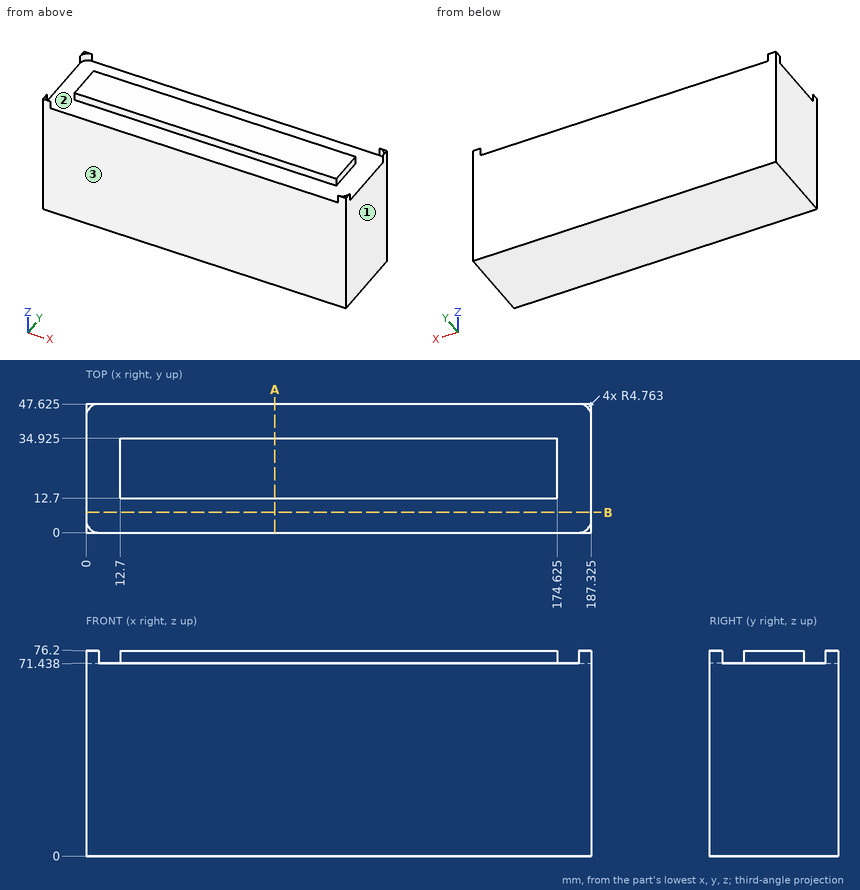
Here's the drawing with two shaded views (mm, measured from the low corner). I have some questions. Round coordinates to 2 decimals unless told otherwise and drop trailing zeros. Loops run counter-clockwise (first coordinate to the right, second up) from the corner with the lowest first, then second, coordinate; pieces in that order, holes last. Notation, with made-up numbers: M 51.25,66.5 L 103.25,66.5 A19 ccw 103.25,91.5 Z; hole C -22.75,5.25 d1. An arc over 180 degrees is marked long. Answer as a JSON object with one key per item and string values. Group by question number.
Q1. Imagine slicing it at B-B, the plane y = 7.5. Please give me the cut outline in (x, z) (1 decimal).
Q2. We'd pull the mould along X, two halves only. Please class the marked faces 1, 2 and 3: +X half, -X half, draft (parallel to the pull), parting line (faces both ways), or undercut.
Q3. Will these pins go through, and if not, where does the flat tip stop? pin 1 (5 mm diameter, centred on y = 23, z = 73.5, fed in from +X) (1 decimal); pin 2 (1.4 mm diameter, centred on x = 113, z = 74, fed in from +Y) (1 decimal); pin 3 (6 mm diameter, centred on x = 82.5, y = 40, fed in from +Z); pin 4 (2.5 mm diameter, centred on x = 118, z = 74.5, fed in from -Y).
Q4. Please list where this line runs through material, in increasing order: L1, parallel to Z at x = 148.5, y = 44.
Q5. Imagine slicing it at A-A, the plane x = 70. Please give me the cut outline in (y, z) (1 decimal), then the cut area to 3 significant figures.
Findings:
{
 "1": {"outline": "M 0,0 L 187.3,0 L 187.3,71.4 L 0,71.4 Z"},
 "2": {"face 1": "+X half", "face 2": "undercut", "face 3": "draft"},
 "3": {"pin 1": "stops at x = 187.3", "pin 2": "stops at y = 34.9", "pin 3": "stops at z = 71.44", "pin 4": "stops at y = 12.7"},
 "4": {"L1": "z = 0 to 71.44"},
 "5": {"outline": "M 0,0 L 47.6,0 L 47.6,71.4 L 34.9,71.4 L 34.9,76.2 L 12.7,76.2 L 12.7,71.4 L 0,71.4 Z", "area": "3,510 mm2"}
}
